Work out the finished part from the listing and answer in its coordinate system (mm). A direction names the side the tool comes from. Round coordinates to 2 decimals unless told otherwise and drop trailing zeros. Write each loop counter-clockwise with the first axis right and the second up, starting at its lowest first coordinate (ties: lowest second). Pieces come first, ordered by that corner, then holes. Notation, with made-up numbers: (4, 51) -> (40, 51) arc R22 ccw to (40, 78) -> close; hole circle Ø8 at (-30.75, 26.5). An arc over 180 degrees is marked (long way). Answer as a JSON object with one key per item and string values. Group by question number.
from build123d import *

# Parameters (mm, degrees)
SKETCH1_R           = 2.2098
BOSS_EXTRUDE1_DEPTH = 6.223
SKETCH2_R           = 4.2164
CUT_EXTRUDE1_DEPTH  = 3.048
SKETCH3_R           = 5.08
CUT_EXTRUDE2_DEPTH  = 2.159
SKETCH4_R           = 4.953
BOSS_EXTRUDE2_DEPTH = 2.032


with BuildPart() as part:
    # Sketch1 → Boss-Extrude1 (new body)
    with BuildSketch(Plane.XY):
        with BuildLine():
            Line((-50.8, -31.75), (50.8, -31.75))
            ThreePointArc((50.8, -31.75), (55.290128061, -29.890128061), (57.15, -25.4))
            Line((57.15, -25.4), (57.15, 25.4))
            ThreePointArc((57.15, 25.4), (55.290128061, 29.890128061), (50.8, 31.75))
            Line((50.8, 31.75), (-50.8, 31.75))
            ThreePointArc((-50.8, 31.75), (-55.290128061, 29.890128061), (-57.15, 25.4))
            Line((-57.15, 25.4), (-57.15, -25.4))
            ThreePointArc((-57.15, -25.4), (-55.290128061, -29.890128061), (-50.8, -31.75))
        make_face()
        with Locations((-50.8, -25.4)):
            Circle(SKETCH1_R, mode=Mode.SUBTRACT)
        with Locations((-50.8, 25.4)):
            Circle(SKETCH1_R, mode=Mode.SUBTRACT)
        with Locations((50.8, 25.4)):
            Circle(SKETCH1_R, mode=Mode.SUBTRACT)
        with Locations((50.8, -25.4)):
            Circle(SKETCH1_R, mode=Mode.SUBTRACT)
    extrude(amount=BOSS_EXTRUDE1_DEPTH)

    # Sketch2 → Cut-Extrude1 (cut)
    with BuildSketch(Plane.XY.offset(6.223)):
        with Locations((-50.8, 25.4)):
            Circle(SKETCH2_R)
        with Locations((50.8, 25.4)):
            Circle(SKETCH2_R)
        with Locations((50.8, -25.4)):
            Circle(SKETCH2_R)
        with Locations((-50.8, -25.4)):
            Circle(SKETCH2_R)
    extrude(amount=-CUT_EXTRUDE1_DEPTH, mode=Mode.SUBTRACT)

    # Sketch3 → Cut-Extrude2 (cut)
    with BuildSketch(Plane.XY.offset(6.223)):
        with Locations((38.1, 0)):
            Circle(SKETCH3_R)
        with Locations((-38.1, 0)):
            Circle(SKETCH3_R)
    extrude(amount=-CUT_EXTRUDE2_DEPTH, mode=Mode.SUBTRACT)

    # Sketch4 → Boss-Extrude2 (add)
    with BuildSketch(Plane.XY.offset(6.223)):
        Circle(SKETCH4_R)
    extrude(amount=BOSS_EXTRUDE2_DEPTH)


solid = part.part
1) A cutting plane is placed at D-D on y = -6.5. Determine the outline of the cut face in (x, z), plus the area to 3 significant figures.
2) Each of these flat-tipped pins is pushed along its axis until it touches: P1, Ø6.5, axis at x = -52.5, y = 23.5, coming from the +Z side; P2, Ø5, axis at x = 50.8, y = 25.4, coming from the +Z side (3 decimals); P3, Ø8, axis at x = -38.1, y = 0, coming from the +Z side; P4, Ø2.5, axis at x = -50, y = -25.5, coming from the +Z side. Where does it stop, or does it pass through?
3) A cutting plane is placed at C-C on x = 38.1. Determine the outline of the cut face in (y, z), plus the area to 3 significant figures.
4) A tool of negligible diameter and unlimited length cuts with its end or side. For faces 1 (the face through (52.91, 26.06, 1.57)), 2 (the face through (34, -3, 5)), from which of +Z, -Z, +X, -X, +Y, -Y can it reach the whole face along a straight path? Write none if from no direction.
5) A cutting plane is placed at B-B on x = 0. Determine the outline of the cut face in (y, z) (3 decimals).
6) Straight lines are drawn through the part: L1, parallel to X at y = -25.4, z = 1.2; L2, parallel to Y at x = -50.8, z = 1.2. For each, find the intervals that lie inside material, in ascending order.
7) For a pull along X with two mould halves and no side action, classify faces 3 (the face through (-53.008, -25.303, 1.565)), 4 (the face through (-55.24, 29.94, 3.07)), 5 (the face through (0, 0, 8.255)) as released by +X, released by -X, zero draft, split by the parting line, or undercut.
8) A cutting plane is placed at A-A on y = 0. Determine the outline of the cut face in (x, z) (3 decimals), plus the area to 3 significant figures.
Established:
{
 "1": {"outline": "(-57.15, 0) -> (57.15, 0) -> (57.15, 6.22) -> (-57.15, 6.22) -> close", "area": "711 mm²"},
 "2": {"P1": "stops at z = 6.22", "P2": "stops at z = 3.175", "P3": "stops at z = 4.06", "P4": "passes through"},
 "3": {"outline": "(-31.75, 0) -> (31.75, 0) -> (31.75, 6.22) -> (5.08, 6.22) -> (5.08, 4.06) -> (-5.08, 4.06) -> (-5.08, 6.22) -> (-31.75, 6.22) -> close", "area": "373 mm²"},
 "4": {"face 1": "+Z, -Z", "face 2": "+Z"},
 "5": {"outline": "(-31.75, 0) -> (31.75, 0) -> (31.75, 6.223) -> (4.953, 6.223) -> (4.953, 8.255) -> (-4.953, 8.255) -> (-4.953, 6.223) -> (-31.75, 6.223) -> close"},
 "6": {"L1": "x = -57.15 to -53.01, -48.59 to 48.59, 53.01 to 57.15", "L2": "y = -31.75 to -27.61, -23.19 to 23.19, 27.61 to 31.75"},
 "7": {"face 3": "undercut", "face 4": "released by -X", "face 5": "zero draft"},
 "8": {"outline": "(-57.15, 0) -> (57.15, 0) -> (57.15, 6.223) -> (43.18, 6.223) -> (43.18, 4.064) -> (33.02, 4.064) -> (33.02, 6.223) -> (4.953, 6.223) -> (4.953, 8.255) -> (-4.953, 8.255) -> (-4.953, 6.223) -> (-33.02, 6.223) -> (-33.02, 4.064) -> (-43.18, 4.064) -> (-43.18, 6.223) -> (-57.15, 6.223) -> close", "area": "688 mm²"}
}
